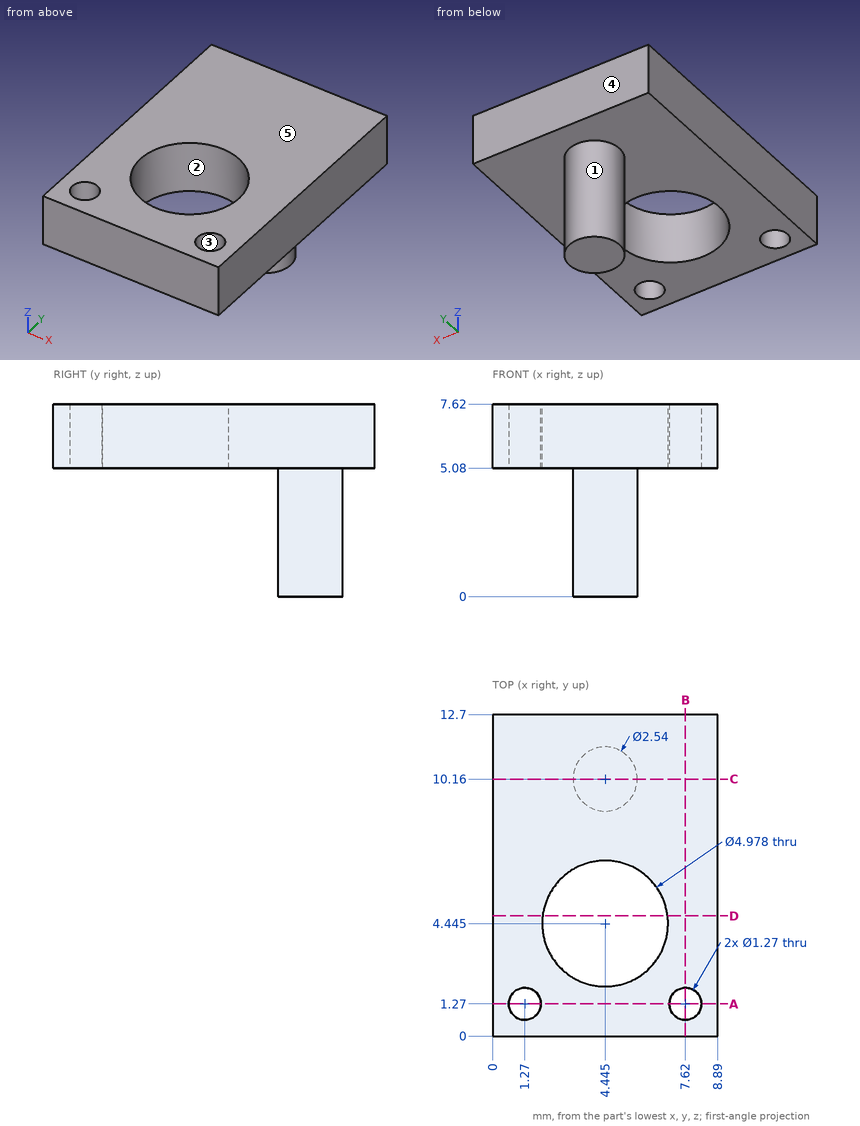
For this review, use the dimensioned drawing (mm, ordinates from the lowest corner) and the shaded views. A direction names the side the tool comes from. Round coordinates to 2 decimals unless told otherwise and drop trailing zeros. Order: outer loops, then holes, each group sorted by start corner. A loop starts at its lowest first (then second) coordinate and runs counter-clockwise, first axis right, second up. Notation, with made-up numbers: (53.5, 71.5) -> (110.5, 71.5) arc R24 cw to (110.5, 109.5) -> close; hole circle Ø7 at (58, 33.5). An arc over 180 degrees is marked (long way). One line per item, written item: value. Start each with the question number.
Q1. Wall thickness on line 1 (X direction, y = 1.27, z = 6.45) (1 decimal); line 2 (Y direction, x = 7.62, z = 7) (1 decimal); line 3 (Z direction, x = 7, y = 4.75): over which ranges is each line inside the solid? List them lowest first.
Q2. Take a section at A-A (y = 1.27). Write out the cut boundary in (x, z) (1 decimal).
Q3. Take a section at D-D (y = 4.75). Write out the cut boundary in (x, z) (1 decimal).
Q4. Clearance check with flat-ended pins moving along their axes: pin 1 Ø2 at (x, y) = (7.62, 1.27) entering from -Z; pin 2 Ø2 at (y, z) = (4, 4.5) entering from -X. State where each tip first meets the part, or that it passes through.
Q5. Take a section at B-B (x = 7.62). Write out the cut boundary in (y, z) (1 decimal).
Q6. Machinability: for the marked faces 1 and 2, which of the approach directions +Z, -Z, +X, -X, +Y, -Y give a long, thin tool a straight path to every point of the face, cutting with its end or side? Answer none if there is none.
Q7. Mouldability with a two-part tool opening along Y and no side actions: class the marked faces 3, 4 and 5 as released by +Y, released by -Y, zero draft, split by the parting line, or undercut.
Q8. Take a section at C-C (y = 10.16). Write out the cut boundary in (x, z) (1 decimal), and give its area (3 significant figures).
Reported:
1. line 1: x = 0 to 0.6, 1.9 to 7, 8.3 to 8.9
1. line 2: y = 0 to 0.6, 1.9 to 12.7
1. line 3: z = 5.08 to 7.62
2. outline: (0, 5.1) -> (0.6, 5.1) -> (0.6, 7.6) -> (0, 7.6) -> close; (1.9, 5.1) -> (7, 5.1) -> (7, 7.6) -> (1.9, 7.6) -> close; (8.3, 5.1) -> (8.9, 5.1) -> (8.9, 7.6) -> (8.3, 7.6) -> close
3. outline: (0, 5.1) -> (2, 5.1) -> (2, 7.6) -> (0, 7.6) -> close; (6.9, 5.1) -> (8.9, 5.1) -> (8.9, 7.6) -> (6.9, 7.6) -> close
4. pin 1: stops at z = 5.08
4. pin 2: stops at x = 0
5. outline: (0, 5.1) -> (0.6, 5.1) -> (0.6, 7.6) -> (0, 7.6) -> close; (1.9, 5.1) -> (12.7, 5.1) -> (12.7, 7.6) -> (1.9, 7.6) -> close
6. face 1: -Z
6. face 2: +Z, -Z
7. face 3: undercut
7. face 4: released by +Y
7. face 5: zero draft
8. outline: (0, 5.1) -> (3.2, 5.1) -> (3.2, 0) -> (5.7, 0) -> (5.7, 5.1) -> (8.9, 5.1) -> (8.9, 7.6) -> (0, 7.6) -> close
8. area: 35.5 mm2
